```python
from build123d import *

# Parameters (mm, degrees)
SKETCH1_R           = 2.0193
SKETCH1_R_2         = 14.2875
BOSS_EXTRUDE1_DEPTH = 3.175
FILLET1_R           = 3.175


with BuildPart() as part:
    # Sketch1 → Boss-Extrude1 (new body)
    with BuildSketch(Plane.XY):
        with BuildLine():
            Line((12.7, -38.1), (12.7, 12.7))
            Line((12.7, 12.7), (-69.85, 12.7))
            ThreePointArc((-69.85, 12.7), (-95.25, -12.7), (-69.85, -38.1))
            Line((-69.85, -38.1), (12.7, -38.1))
        make_face()
        Circle(SKETCH1_R, mode=Mode.SUBTRACT)
        with Locations((0, -12.7)):
            Circle(SKETCH1_R, mode=Mode.SUBTRACT)
        with Locations((0, -25.4)):
            Circle(SKETCH1_R, mode=Mode.SUBTRACT)
        with Locations((-69.85, -12.7)):
            Circle(SKETCH1_R_2, mode=Mode.SUBTRACT)
    extrude(amount=BOSS_EXTRUDE1_DEPTH)

    # Fillet1
    fillet1_edges = [part.edges().sort_by_distance(p)[0] for p in [
        (12.7, 12.7, 1.5875),
        (12.7, -38.1, 1.5875),
    ]]
    fillet(fillet1_edges, radius=FILLET1_R)


solid = part.part
```
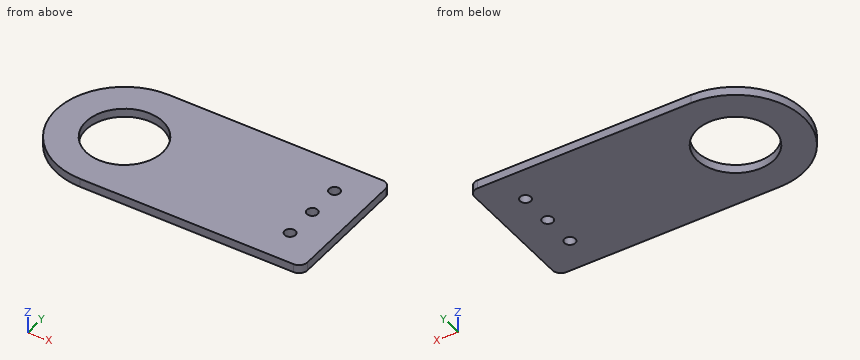
The listing builds one solid part. Answer for the finished solid, in the listing's coordinates (mm). Round coordinates to 2 decimals unless told otherwise and drop trailing zeros. Loops run counter-clockwise (first coordinate to the right, second up) from the corner with the lowest first, then second, coordinate; pieces in that order, holes last. Notation, with made-up numbers: (-11.5, 36) - (6.5, 36) arc R16 ccw to (6.5, 56) - close; hole circle Ø1 at (-0.75, 85.5). An arc over 180 degrees is marked (long way). Return JSON: item names as keys, results as strings. Group by question number.
1. Consider probe 1 along Y at (x, z) = (0, 0.7); probe 2 along Y at (x, z) = (-69.85, 1.25); probe 3 along Y at (x, z) = (-61, 0.8). Determine where each line is inside the solid, lowest interval first.
2. Each of these flat-tipped pins is pushed along its axis until it touches: P1, Ø1, axis at y = 3, z = 2.5, coming from the -X side; P2, Ø17, axis at x = -69.85, y = -12.7, coming from the +Z side; P3, Ø1, axis at y = 5, z = 2.5, coming from the -X side. Where does it stop, or does it pass through?
3. The part is cut by section A-A on x = 0. Determine the outline of the cut face in (y, z) (3 decimals).
4. The part is cut by section B-B on y = -12.7. State how many separate pieces and enclosed holes the cut face has, then the cut area to 3 significant figures.
5. The part is cut by section D-D on y = -1. Determine the outline of the cut face in (x, z) (3 decimals).
Resolved:
{
 "1": {"probe 1": "y = -38.1 to -27.42, -23.38 to -14.72, -10.68 to -2.02, 2.02 to 12.7", "probe 2": "y = -38.1 to -26.99, 1.59 to 12.7", "probe 3": "y = -38.1 to -23.92, -1.48 to 12.7"},
 "2": {"P1": "stops at x = -90.2", "P2": "passes through", "P3": "stops at x = -88.54"},
 "3": {"outline": "(-38.1, 0) - (-27.419, 0) - (-27.419, 3.175) - (-38.1, 3.175) - close; (-23.381, 0) - (-14.719, 0) - (-14.719, 3.175) - (-23.381, 3.175) - close; (-10.681, 0) - (-2.019, 0) - (-2.019, 3.175) - (-10.681, 3.175) - close; (2.019, 0) - (12.7, 0) - (12.7, 3.175) - (2.019, 3.175) - close"},
 "4": {"separate pieces": "3", "enclosed holes": "0", "area": "239 mm²"},
 "5": {"outline": "(-92.395, 0) - (-78.05, 0) - (-78.05, 3.175) - (-92.395, 3.175) - close; (-61.65, 0) - (-1.754, 0) - (-1.754, 3.175) - (-61.65, 3.175) - close; (1.754, 0) - (12.7, 0) - (12.7, 3.175) - (1.754, 3.175) - close"}
}
